Verification items for the finished model (mm, model axes). A direction names the side the tool comes from. Give positions to 0.01 mm unless a question says otherwise; leave off trailing zeros. Order: outer loops, then holes, each group sorted by start corner. A loop starts at its lowest first (then second) coordinate and runs counter-clockwise, first axis right, second up.
(1) Mould release check, pull along X, two halves, no side actions. Record for faces 3 (the face through (-11, 0, 37)), 4 (the face through (-10.59, -0.55, 42.71)), 5 (the face through (11, 0, 34)), 6 (the face through (0, 0, 0.2)): pulls with the +X half, pulls with the -X half, needs draft (parallel to the pull), parting line crosses it, or undercut.
(2) Gauge pin test, flat ends, axial feed: pin 1 (1 mm diameter, centred on x = 7.5, y = -9.5, fed in from +Z); pin 2 (4 mm diameter, centred on y = 1, z = 35, fed in from +X); pin 3 (0.6 mm diameter, centred on x = -10.5, z = 34, fed in from +Y). Record the tip position at first contact, or that the pin passes through.
(3) Sectioned sample at C-C on x = 0. Record the cut outline in (y, z), plus the area to 3 significant figures.
(4) Sectioned sample at A-A on y = 0. Record the cut outline in (x, z).
(5) Scan lines: L1, parallel to Y at x = -10.75, z = 42; L2, parallel to X at y = -3.5, z = 37; L3, parallel to Z at x = 9.5, y = -5.25. Record each from-to range of solid material in increasing order.
(6) Sectioned sample at B-B on z = 42. Record the cut outline in (x, y).
(7) Sectioned sample at D-D on z = 28.5. Record the cut outline in (x, y), plus the area to 3 significant figures.
(8) Access from +Z, -Z, +X, -X, +Y, -Y to the whole of each face (thin tool, end or side, straight path). Record for faces 1 (the face through (-10.6, -2.5, 45.2)), 2 (the face through (10.2, 0, 34)).
Autodesk Inventor part; units mm, degrees
ref_plane "YZ Plane" through (0, 0, 0) normal (1, 0, 0) x (0, 1, 0)
ref_plane "XZ Plane" through (0, 0, 0) normal (0, 1, 0) x (-1, 0, 0)
ref_plane "XY Plane" through (0, 0, 0) normal (0, 0, 1) x (1, 0, 0)
sketch "Skizze1" plane through (0, 0, 0) normal (0, 0, 1) x (1, 0, 0)
  circle A0 centre (0, 0) radius 13.1
  dimension "d0" = 26.2
extrude "Extrusion1" add sketch "Skizze1" along normal blind 29
sketch "Skizze2" plane through (0, 0, 29) normal (0, 0, 1) x (1, 0, 0)
  line L0 (-11, 3.75) -> (-10.2, 3.75)
  line L1 (-10.2, 3.75) -> (-10.2, -3.75)
  line L2 (-10.2, -3.75) -> (-11, -3.75)
  line L3 (-11, -3.75) -> (-11, 3.75)
  line L4 (10.2, 3.75) -> (11, 3.75)
  line L5 (11, 3.75) -> (11, -3.75)
  line L6 (11, -3.75) -> (10.2, -3.75)
  line L7 (10.2, -3.75) -> (10.2, 3.75)
  line L8 (10.2, 0) -> (-10.2, 0) construction
  point P0 (0, 0)
  point P1 (0, 0)
  dimension "d3" = 7.5
  dimension "d4" = 0.8
  dimension "d6" = 22
sketch "Skizze3" plane through (0, 0, 0) normal (0, 1, 0) x (-1, 0, 0)
  line L0 (13.1, 29) -> (-13.1, 29)
  line L1 (-13.1, 0) -> (13.1, 0)
  line L2 (-13.1, 0) -> (-13.1, 29)
  line L3 (13.1, 0) -> (13.1, 29)
  point P0 (0, 0)
  dimension "d7" = 29
extrude "Extrusion2" add sketch "Skizze2" along normal blind 17
sketch "Skizze4" plane through (11, -3.75, 29) normal (1, 0, 0) x (0, 0, -1)
  line L0 (0, 7.5) -> (0, 0)
  line L1 (0, 7.5) -> (-17, 7.5) construction
  line L2 (-17, 0) -> (-17, 7.5) construction
  line L3 (0, 0) -> (-17, 0) construction
  line L4 (0, 0) -> (-17, 0) construction
  line L5 (-9, 0) -> (-9, 0.55)
  line L6 (-9, 0.55) -> (-15.5, 0.55)
  line L7 (-15.5, 0.55) -> (-17, 2.05)
  line L8 (-17, 5.45) -> (-15.5, 6.95)
  line L9 (-15.5, 6.95) -> (-9, 6.95)
  line L10 (-9, 6.95) -> (-9, 7.5)
  line L11 (0, 7.5) -> (-17, 7.5) construction
  circle A0 centre (-13, 3.75) radius 0.9
  line L12 (-13, 3.75) -> (-17, 3.75) construction
  line L13 (-17, 0) -> (-17, 7.5) construction
  line L14 (-17, 0) -> (-17, 7.5) construction
  line L15 (-9, 0) -> (-17, 0)
  line L16 (-17, 2.05) -> (-17, 0)
  line L17 (-17, 5.45) -> (-17, 7.5)
  line L18 (-9, 7.5) -> (-17, 7.5)
  point P0 (29, 3.75)
  dimension "d10" = 45
  dimension "d11" = 45
  dimension "d12" = 6.4
  dimension "d13" = 8
  dimension "d14" = 1.5
  dimension "d15" = 1.8
  dimension "d16" = 4
extrude "Extrusion3" cut sketch "Skizze4" against normal through all
sketch "Skizze5" plane through (0, 0, 0) normal (0, 0, -1) x (-1, 0, 0)
  line L0 (-3, 2) -> (3, 2)
  line L1 (3, 2) -> (3, -2)
  line L2 (3, -2) -> (-3, -2)
  line L3 (-3, -2) -> (-3, 2)
  line L4 (3, -2) -> (-3, 2) construction
  point P0 (0, 0)
  point P1 (0, 0)
  dimension "d19" = 6
  dimension "d20" = 4
extrude "Extrusion4" cut sketch "Skizze5" against normal blind 0.2
sketch "Skizze6" plane through (11, -3.75, 29) normal (1, 0, 0) x (0, 0, -1)
  line L0 (-17, 7.5187) -> (-11, 7.5187)
  line L1 (-11, 7.5187) -> (-11, -0.0187)
  line L2 (-11, -0.0187) -> (-17, -0.0187)
  line L3 (-17, -0.0187) -> (-17, 7.5187)
  line L4 (-17, 2.05) -> (-17, 5.45)
  point P0 (29, 3.75)
  point P1 (-17, 3.75)
  dimension "d23" = 6
extrude "Extrusion5" cut sketch "Skizze6" against normal blind 1
equation "\"d11\" = d10"
properties part number "Zündspule"
Ans:
1. face 3: pulls with the -X half
1. face 4: needs draft
1. face 5: pulls with the +X half
1. face 6: undercut
2. pin 1: stops at z = 29
2. pin 2: stops at x = 11
2. pin 3: stops at y = 3.75
3. outline: (-13.1, 0) - (-2, 0) - (-2, 0.2) - (2, 0.2) - (2, 0) - (13.1, 0) - (13.1, 29) - (-13.1, 29) - close
3. area: 759 mm2
4. outline: (-13.1, 0) - (-3, 0) - (-3, 0.2) - (3, 0.2) - (3, 0) - (13.1, 0) - (13.1, 29) - (11, 29) - (11, 40) - (10.2, 40) - (10.2, 29) - (-10.2, 29) - (-10.2, 41.1) - (-11, 41.1) - (-11, 29) - (-13.1, 29) - close; (-11, 42.9) - (-10.2, 42.9) - (-10.2, 46) - (-11, 46) - close
5. L1: y = -3.2 to -0.9, 0.9 to 3.2
5. L2: x = -11 to -10.2, 10.2 to 11
5. L3: z = 0 to 29
6. outline: (-11, -3.2) - (-10.2, -3.2) - (-10.2, -0.9) - (-11, -0.9) - close; (-11, 0.9) - (-10.2, 0.9) - (-10.2, 3.2) - (-11, 3.2) - close
7. outline: circle Ø26.2 at (0, 0)
7. area: 539 mm2
8. face 1: +Z, +X, -X, -Y
8. face 2: +Z, +Y, -Y
